Read the model definition and answer for the solid it produces. Units are mm, in the model's axes. Face numbers are marked on the shaded views. A direction names the side the tool comes from. Round coordinates to 2 decimals unless told otherwise and drop trailing zeros. Order: outer loops, then holes, each group sorted by start corner. A loop starts at its lowest first (then second) coordinate and runs counter-clockwise, first axis right, second up. Notation, with made-up numbers: (19, -10.75) - (61, -10.75) arc R8 cw to (61, 0.25) - close; hole circle Ø3 at (11.5, -4). An arc over 180 degrees is marked (long way). Put each result on its own line as item: value. Start each with the question number.
Q1. For a pull along Y with two mould halves and no side action, classify the marked faces 5, 6 and 7 as pulls with the +Y half, pulls with the -Y half, needs draft (parallel to the pull), parting line crosses it, or undercut.
Q2. Section A-A on z = 2.25 is taken. Give the vertices of the cut face in (x, y) (3 decimals), then the cut area to 3 significant figures.
Q3. Which of the six approach directions +Z, -Z, +X, -X, +Y, -Y give full straight-line access (tool end or side, diameter ignored) to the marked faces 1, 2, 3 and 4?
Q4. Find the intervals of material crossed by line 1 along X through (y, z) = (4.5, 3.25); line 2 along X through (y, z) = (1.75, 6.75); line 3 along Y through (x, z) = (3, 4.5), in increasing order. Write a range as from..to.
Q5. Each of these flat-tipped pins is pushed along its axis until it touches: pin 1 Ø1 at (x, z) = (4.5, 4.5) entering from -Y (3 decimals); pin 2 Ø3 at (y, z) = (3.5, 4) entering from +X; pin 3 Ø2 at (y, z) = (3.5, 7) entering from -X. Where does it stop, or does it pass through?
Q6. Section D-D on x = 0.25 is taken. Give the vertices of the cut face in (y, z).
Q7. Section C-C on y = 7.62 is taken. Give the vertices of the cut face in (x, z), then the cut area to 3 significant figures.
Q8. Section B-B on x = 3 is taken. Give the vertices of the cut face in (y, z), then the cut area to 3 significant figures.
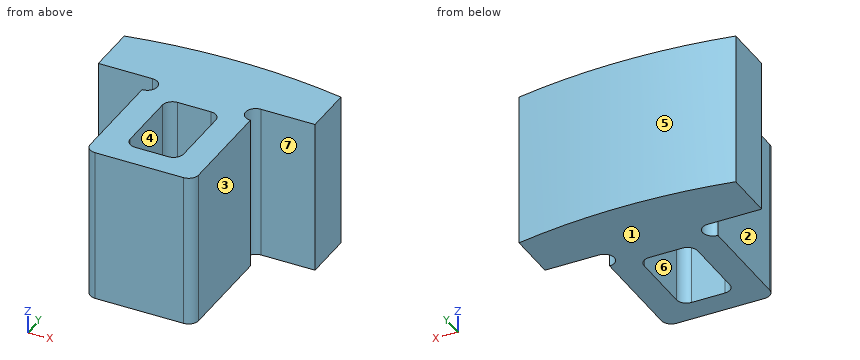
from build123d import *

# Parameters (mm, degrees)
F1_DEPTH = 9.779


with BuildPart() as f1:
    # F0 (on Top) → F1 (new body)
    with BuildSketch(Plane.XY):
        with BuildLine():
            ThreePointArc((-3.429, 0.635), (-3.243013, 0.185987), (-2.794, 0))
            Line((-2.794, 0), (2.794, 0))
            ThreePointArc((2.794, 0), (3.243013, 0.185987), (3.429, 0.635))
            Line((3.429, 0.635), (3.429, 6.985))
            ThreePointArc((3.429, 6.985), (2.794, 7.62), (3.429, 8.255))
            Line((3.429, 8.255), (6.858, 8.255))
            Line((6.858, 8.255), (6.858, 11.43))
            ThreePointArc((6.858, 11.43), (0, 12.065), (-6.858, 11.43))
            Line((-6.858, 11.43), (-6.858, 8.255))
            Line((-6.858, 8.255), (-3.429, 8.255))
            ThreePointArc((-3.429, 8.255), (-2.794, 7.62), (-3.429, 6.985))
            Line((-3.429, 6.985), (-3.429, 0.635))
        make_face()
        with BuildLine():
            ThreePointArc((-1.6891, 6.096), (-1.503113, 6.545013), (-1.0541, 6.731))
            Line((-1.0541, 6.731), (1.0541, 6.731))
            ThreePointArc((1.0541, 6.731), (1.503113, 6.545013), (1.6891, 6.096))
            Line((1.6891, 6.096), (1.6891, 2.159))
            ThreePointArc((1.6891, 2.159), (1.503113, 1.709987), (1.0541, 1.524))
            Line((1.0541, 1.524), (-1.0541, 1.524))
            ThreePointArc((-1.0541, 1.524), (-1.503113, 1.709987), (-1.6891, 2.159))
            Line((-1.6891, 2.159), (-1.6891, 6.096))
        make_face(mode=Mode.SUBTRACT)
    extrude(amount=F1_DEPTH)


solid = f1.part
Findings:
1. face 5: pulls with the +Y half
1. face 6: undercut
1. face 7: pulls with the -Y half
2. outline: (-6.858, 8.255) - (-3.429, 8.255) arc R0.635 cw to (-3.429, 6.985) - (-3.429, 0.635) arc R0.635 ccw to (-2.794, 0) - (2.794, 0) arc R0.635 ccw to (3.429, 0.635) - (3.429, 6.985) arc R0.635 cw to (3.429, 8.255) - (6.858, 8.255) - (6.858, 11.43) arc R37.351 ccw to (-6.858, 11.43) - close; hole (-1.689, 2.159) arc R0.635 ccw to (-1.054, 1.524) - (1.054, 1.524) arc R0.635 ccw to (1.689, 2.159) - (1.689, 6.096) arc R0.635 ccw to (1.054, 6.731) - (-1.054, 6.731) arc R0.635 ccw to (-1.689, 6.096) - close
2. area: 87.3 mm2
3. face 1: -Z, +X, -X, +Y, -Y
3. face 2: +Z, -Z, -X, -Y
3. face 3: +Z, -Z, +X, -Y
3. face 4: +Z, -Z
4. line 1: -3.43..-1.69, 1.69..3.43
4. line 2: -3.43..-1.54, 1.54..3.43
4. line 3: 0.03..7.15, 8.09..11.94
5. pin 1: y = 8.255
5. pin 2: x = 3.43
5. pin 3: x = -3.43
6. outline: (0, 0) - (1.52, 0) - (1.52, 9.78) - (0, 9.78) - close; (6.73, 0) - (12.06, 0) - (12.06, 9.78) - (6.73, 9.78) - close
7. outline: (-2.79, 0) - (2.79, 0) - (2.79, 9.78) - (-2.79, 9.78) - close
7. area: 54.6 mm2
8. outline: (0.03, 0) - (7.15, 0) - (7.15, 9.78) - (0.03, 9.78) - close; (8.09, 0) - (11.94, 0) - (11.94, 9.78) - (8.09, 9.78) - close
8. area: 107 mm2
